Verification items for the finished model (mm, model axes). Face numbers are marked on the shaded views. A direction names the side the tool comes from. Coordinates: 2 decimals unless noted, no trailing zeros. Write each loop counter-clockwise with the first axis right and the second up, starting at its lowest first coordinate (ties: lowest second). Pieces come first, ordered by that corner, then holes. Notation, with made-up numbers: (86, 41.25) -> (105, 41.25) arc R24 ccw to (105, 52.25) -> close; hole circle Ø2 at (83.25, -35.75). An arc over 180 degrees is marked (long way). Answer in a Markdown table with one row per item.
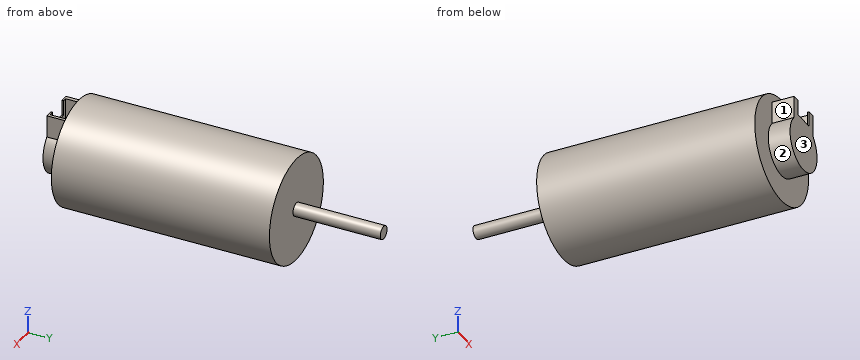
```python
from build123d import *

# Parameters (mm, degrees)
SKETCH1_R           = 12
BOSS_EXTRUDE1_DEPTH = 50
SKETCH2_R           = 1.5
BOSS_EXTRUDE2_DEPTH = 20
BOSS_EXTRUDE3_DEPTH = 5
SKETCH4_W           = 7
SKETCH4_H           = 4
CUT_EXTRUDE1_DEPTH  = 5
SKETCH5_W           = 5
SKETCH5_H           = 3.450611601
CUT_EXTRUDE2_DEPTH  = 0.4


with BuildPart() as part:
    # Sketch1 → Boss-Extrude1 (new body)
    with BuildSketch(Plane(origin=(0, 0, 0), x_dir=(1, 0, 0), z_dir=(0, 1, 0))):
        with Locations(Location((0, 0, 0), (0, 0, 270))):
            Circle(SKETCH1_R)
    extrude(amount=BOSS_EXTRUDE1_DEPTH)

    # Sketch2 → Boss-Extrude2 (add)
    with BuildSketch(Plane(origin=(0, 50, 0), x_dir=(1, 0, 0), z_dir=(0, 1, 0))):
        with Locations(Location((0, 0, 0), (0, 0, 270))):
            Circle(SKETCH2_R)
    extrude(amount=BOSS_EXTRUDE2_DEPTH)

    # Sketch3 → Boss-Extrude3 (add)
    with BuildSketch(Plane.XZ):
        with BuildLine():
            Line((-4.284272991, 4.200595784), (-4.284272991, 9.25435285))
            Line((-4.284272991, 9.25435285), (4.284272991, 9.25435285))
            Line((4.284272991, 9.25435285), (4.284272991, 4.200595784))
            ThreePointArc((4.284272991, 4.200595784), (0, -6), (-4.284272991, 4.200595784))
        make_face()
    extrude(amount=BOSS_EXTRUDE3_DEPTH)

    # Sketch4 → Cut-Extrude1 (cut)
    with BuildSketch(Plane.XY.offset(9.25435285)):
        with Locations((0.08918727, -2.633127674)):
            Rectangle(SKETCH4_W, SKETCH4_H)
    extrude(amount=-CUT_EXTRUDE1_DEPTH, mode=Mode.SUBTRACT)

    # Sketch5 → Cut-Extrude2 (cut)
    with BuildSketch(Plane.XZ.offset(5)):
        with Locations((-0.001847359, 7.52904705)):
            Rectangle(SKETCH5_W, SKETCH5_H)
    extrude(amount=-CUT_EXTRUDE2_DEPTH, mode=Mode.SUBTRACT)


solid = part.part
```
1. Sectioned sample at A-A, the plane x = 0. Record the cut outline in (y, z).
Findings below:
| item | result |
|---|---|
| outline | (-5, -6) -> (0, -6) -> (0, -12) -> (50, -12) -> (50, -1.5) -> (70, -1.5) -> (70, 1.5) -> (50, 1.5) -> (50, 12) -> (0, 12) -> (0, 9.25) -> (-0.63, 9.25) -> (-0.63, 4.25) -> (-4.63, 4.25) -> (-4.63, 5.8) -> (-5, 5.8) -> close |
2. Sectioned sample at D-D, the plane x = -5. Record the cut outline in (y, z), and give its area (3 significant figures).
Findings below:
| item | result |
|---|---|
| outline | (-5, -3.32) -> (0, -3.32) -> (0, -10.91) -> (50, -10.91) -> (50, 10.91) -> (0, 10.91) -> (0, 3.32) -> (-5, 3.32) -> close |
| area | 1,120 mm² |
3. Sectioned sample at C-C, the plane y = 29. Record the cut outline in (x, z).
Findings below:
| item | result |
|---|---|
| outline | circle Ø24 at (0, 0) |
4. Material ranges on probe 1 along Y at (x, z) = (0.75, 4.5); probe 2 along Y at (x, z) = (7.5, 2.5); probe 3 along Y at (x, z) = (-2, 3.25), recorded low to high. Write a range as from..to.
Findings below:
| item | result |
|---|---|
| probe 1 | y = -5..-4.63, -0.63..50 |
| probe 2 | y = 0..50 |
| probe 3 | y = -5..50 |
5. Sectioned sample at B-B, the plane z = 0. Record the cut outline in (x, y), and give its area (3 significant figures).
Findings below:
| item | result |
|---|---|
| outline | (-12, 0) -> (-6, 0) -> (-6, -5) -> (6, -5) -> (6, 0) -> (12, 0) -> (12, 50) -> (1.5, 50) -> (1.5, 70) -> (-1.5, 70) -> (-1.5, 50) -> (-12, 50) -> close |
| area | 1,320 mm² |
6. Go/stop test with flat-tipped pins: pin 1 (3 mm diameter, centred on y = -2.5, z = 6, fed in from +X); pin 2 (1.5 mm diameter, centred on y = 7.5, z = -4, fed in from -X); pin 3 (5.5 mm diameter, centred on y = -3.5, z = 7, fed in from -X). Record where each tip stops, or that it passes through.
Findings below:
| item | result |
|---|---|
| pin 1 | stops at x = 4.28 |
| pin 2 | stops at x = -11.55 |
| pin 3 | stops at x = -4.28 |
7. Access from +Z, -Z, +X, -X, +Y, -Y to the whole of each face (thin tool, end or side, straight path). Record for the marked faces 1, 2 and 3.
Findings below:
| item | result |
|---|---|
| face 1 | +Z, -X, -Y |
| face 2 | -Y |
| face 3 | +Z, -Z, +X, -X, -Y |
